Input: part model. Units: mm. Frame: model coordinates. Face numbers are marked on the shaded views. A direction names the side the tool comes from. Coordinates: 2 decimals unless noted, no trailing zeros. Order: outer loops, then holes, each group sorted by start corner. A loop starts at its lowest first (then second) coordinate and runs counter-clockwise, first axis right, second up. Notation, with made-up numbers: (-7, 33) -> (26, 33) arc R29 ccw to (26, 68) -> close; hole circle Ø7 at (14, 54.5). An arc over 180 degrees is marked (long way). Use one line per item in the form item = value. Start each with the question number.
1) Section query B-B on x = 18.5. Output: boundary loops of the cut face in (y, z).
2) Access query for the marked faces 1, 2, 3, 4 and 5. Directions: +Z, -Z, +X, -X, +Y, -Y. A direction counts if a zero-diameter tool reaches every point of the face in a straight line with its end or side. Return the directions, or none.
3) Section query D-D on y = 15.5. Output: boundary loops of the cut face in (x, z).
4) Section query C-C on y = 5. Output: boundary loops of the cut face in (x, z), then the cut area to 3 significant figures.
5) Pin query (flat end, axial travel): pin 1 (6 mm diameter, centred on x = 3.5, z = -15.5, fed in from -Y); pin 2 (3 mm diameter, centred on x = 0, y = 5, fed in from -Z); pin 3 (2 mm diameter, centred on y = 2, z = 3, fed in from +X); pin 4 (2.5 mm diameter, centred on y = 5, z = 0, fed in from +X). Return the tip coordinate at first contact, or that it passes through.
6) Ray query, line 1 along Y through (x, z) = (0, 2); line 2 along Y through (x, z) = (30.5, -28); line 3 along Z through (x, y) = (2, 5.5). Return the intervals inside material, ascending.
7) Section query A-A on z = 0. Output: boundary loops of the cut face in (x, y), then the cut area to 3 significant figures.
8) Draft query along X for the marked faces 6, 7 and 8. Return one class per face: pulls with the +X half, pulls with the -X half, needs draft (parallel to the pull), parting line crosses it, or undercut.
from build123d import *

# Parameters (mm, degrees)
SKETCH1_W           = 10
SKETCH1_H           = 10
BOSS_EXTRUDE1_DEPTH = 10
SKETCH2_R           = 1.6
CUT_EXTRUDE1_DEPTH  = 3.2
SKETCH3_R           = 1.6
CUT_EXTRUDE3_DEPTH  = 3.2
SKETCH4_R           = 1.6
CUT_EXTRUDE4_DEPTH  = 3.2
FILLET2_R           = 1
CHAMFER1_SIZE       = 6
BOSS_EXTRUDE2_DEPTH = 50
SKETCH6_R           = 1.475
CUT_EXTRUDE5_DEPTH  = 4.1
FILLET3_R           = 0.5
FILLET4_R           = 50


with BuildPart() as part:
    # Sketch1 → Boss-Extrude1 (new body)
    with BuildSketch(Plane(origin=(0, 0, 0), x_dir=(1, 0, 0), z_dir=(0, 1, 0))):
        Rectangle(SKETCH1_W, SKETCH1_H)
    extrude(amount=BOSS_EXTRUDE1_DEPTH)

    # Sketch2 → Cut-Extrude1 (cut)
    with BuildSketch(Plane.XY.offset(5)):
        with Locations((0, 5)):
            Circle(SKETCH2_R)
    extrude(amount=-CUT_EXTRUDE1_DEPTH, mode=Mode.SUBTRACT)

    # Sketch3 → Cut-Extrude3 (cut)
    with BuildSketch(Plane(origin=(0, 0, 0), x_dir=(-1, 0, 0), z_dir=(0, -1, 0))):
        with Locations(Location((0, 0, 0), (0, 0, 90))):
            Circle(SKETCH3_R)
    extrude(amount=-CUT_EXTRUDE3_DEPTH, mode=Mode.SUBTRACT)

    # Sketch4 → Cut-Extrude4 (cut)
    with BuildSketch(Plane(origin=(-5, 0, 0), x_dir=(0, 0, -1), z_dir=(1, 0, 0))):
        with Locations((0, 5)):
            Circle(SKETCH4_R)
    extrude(amount=CUT_EXTRUDE4_DEPTH, mode=Mode.SUBTRACT)

    # Fillet2
    fillet2_edges = [part.edges().sort_by_distance(p)[0] for p in [
        (0, 0, 5),
        (-5, 0, 0),
        (-5, 5, 5),
    ]]
    fillet(fillet2_edges, radius=FILLET2_R)

    # Chamfer1
    chamfer1_edges = [part.edges().sort_by_distance(p)[0] for p in [
        (5, 10, 0),
        (5, 5, -5),
        (0, 10, -5),
    ]]
    chamfer(chamfer1_edges, length=CHAMFER1_SIZE)

    # Sketch5 → Boss-Extrude2 (add)
    with BuildSketch(Plane(origin=(2.666666667, 2.666666667, -2.666666667), x_dir=(-0.4082482904638649, -0.4082482904638639, -0.8164965809277248), z_dir=(0.5773502691896257, 0.577350269189624, -0.5773502691896276))):
        Polygon((0.40824829, 4.949747468), (-2.041241452, 6.363961031), (-4.490731195, 4.949747468), (-4.490731195, 2.121320344), (-2.041241452, 0.707106781), (0.40824829, 2.121320344), align=None)
    extrude(amount=BOSS_EXTRUDE2_DEPTH)

    # Sketch13 → Loft3 section 0
    with BuildSketch(Plane(origin=(25.760677434, 25.760677434, -25.760677434), x_dir=(-0.8164965809277259, 0.4082482904638619, -0.4082482904638644), z_dir=(0.577350269189626, 0.577350269189624, -0.5773502691896274))):
        with BuildLine():
            Line((2.041241452, 6.363961031), (-0.40824829, 4.949747468))
            Line((-0.40824829, 4.949747468), (-0.40824829, 2.121320344))
            Line((-0.40824829, 2.121320344), (2.041241452, 0.707106781))
            Line((2.041241452, 0.707106781), (4.490731195, 2.121320344))
            Line((4.490731195, 2.121320344), (4.490731195, 4.949747468))
            Line((4.490731195, 4.949747468), (2.041241452, 6.363961031))
        make_face()
    # Sketch12 → Loft3 section 1
    with BuildSketch(Plane(origin=(31.534180126, 31.534180126, -31.534180126), x_dir=(-0.40824829046386485, -0.4082482904638636, -0.8164965809277249), z_dir=(0.577350269189626, 0.5773502691896241, -0.5773502691896275))):
        with BuildLine():
            Line((1.40824829, 1.543970074), (1.40824829, 5.527097737))
            Line((1.40824829, 5.527097737), (-2.041241452, 7.518661569))
            Line((-2.041241452, 7.518661569), (-5.490731195, 5.527097737))
            Line((-5.490731195, 5.527097737), (-5.490731195, 1.543970074))
            Line((-5.490731195, 1.543970074), (-2.041241452, -0.447593757))
            Line((-2.041241452, -0.447593757), (1.40824829, 1.543970074))
        make_face()
    loft()

    # Sketch6 → Cut-Extrude5 (cut)
    with BuildSketch(Plane(origin=(31.534180126, 31.534180126, -31.534180126), x_dir=(-0.40824829046386507, -0.4082482904638639, -0.8164965809277246), z_dir=(0.5773502691896257, 0.5773502691896238, -0.5773502691896278))):
        with Locations(Location((-2.041241452, 3.535533906, 0), (0, 0, 30))):
            Circle(SKETCH6_R)
    extrude(amount=-CUT_EXTRUDE5_DEPTH, mode=Mode.SUBTRACT)

    # Fillet3
    fillet3_edges = [part.edges().sort_by_distance(p)[0] for p in [
        (28.459265169, 37.68401004, -28.459265169),
        (31.27576175, 36.27576175, -27.051016879),
        (32.68401004, 33.459265169, -28.459265169),
        (31.27576175, 32.051016879, -31.27576175),
        (28.459265169, 33.459265169, -32.68401004),
        (27.051016879, 36.27576175, -31.27576175),
    ]]
    fillet(fillet3_edges, radius=FILLET3_R)

    # Fillet4
    # the kernel refuses this fillet: 50 mm, written as the material it adds along each edge
    with BuildSketch(Plane(origin=(30.502434506, 27.094010768, -19.685587029), x_dir=(0.6151072128065446, 0.49324054325118827, -0.6151072128065457), z_dir=(-0.7071067811865475, -1.8318679906315083e-15, -0.7071067811865477))) as fillet4_piece_1_section:
        with BuildLine():
            CenterArc((FILLET4_R * 0.0498756211209, FILLET4_R), FILLET4_R, 264.289406863, 5.710593137)
            Line((-FILLET4_R * 0.0496280979001, FILLET4_R * 0.00496280979001), (0, 0))
            Line((0, 0), (FILLET4_R * 0.0498756211209, 0))
        make_face()
    fillet4_piece_1 = extrude(amount=15.297332405, mode=Mode.PRIVATE)
    fillet4_piece_1 = fillet4_piece_1 - Plane(origin=(5.44602295, 2.037599211, -65.47905465), x_dir=(0.4636707308133369, 0.463670730813339, 0.7549959647402431), z_dir=(0.7071067811865475, -0.7071067811865478, 2.220446049250313e-15)) * Cylinder(50, 41, mode=Mode.PRIVATE)
    fillet4_piece_1 = fillet4_piece_1 - Plane(origin=(65.47905465, 7.44602295, -0.037599211), x_dir=(-0.7549959647402456, 0.4636707308133344, -0.46367073081333715), z_dir=(0, 0.7071067811865497, 0.7071067811865455)) * Cylinder(50, 41, mode=Mode.PRIVATE)
    add(fillet4_piece_1)
    with BuildSketch(Plane(origin=(26.094010768, 33.502434506, -17.685587029), x_dir=(0.6557294359916664, 0.5338627664363041, -0.5338627664363074), z_dir=(0, -0.7071067811865497, -0.7071067811865455))) as fillet4_piece_2_section:
        with BuildLine():
            CenterArc((FILLET4_R * 0.0498756211209, FILLET4_R), FILLET4_R, 264.289406863, 5.710593137)
            Line((-FILLET4_R * 0.0496280979001, FILLET4_R * 0.00496280979001), (0, 0))
            Line((0, 0), (FILLET4_R * 0.0498756211209, 0))
        make_face()
    fillet4_piece_2 = extrude(amount=15.297332405, mode=Mode.PRIVATE)
    fillet4_piece_2 = fillet4_piece_2 - Plane(origin=(42.862428257, 50.270851996, 20.170603443), x_dir=(-0.3487737328890522, -0.34877373288905417, -0.8698929626645284), z_dir=(-0.7071067811865471, 0.7071067811865479, -1.8596235662471372e-15)) * Cylinder(50, 41, mode=Mode.PRIVATE)
    fillet4_piece_2 = fillet4_piece_2 - Plane(origin=(48.270851996, -15.170603443, -39.862428257), x_dir=(-0.34877373288905117, 0.8698929626645311, 0.3487737328890489), z_dir=(0.7071067811865476, 1.831867990631508e-15, 0.7071067811865476)) * Cylinder(50, 41, mode=Mode.PRIVATE)
    add(fillet4_piece_2)
    with BuildSketch(Plane(origin=(19.685587029, 35.502434506, -22.094010768), x_dir=(0.6151072128065466, 0.6151072128065448, -0.49324054325118677), z_dir=(0.7071067811865472, -0.7071067811865479, 1.7763568394002505e-15))) as fillet4_piece_3_section:
        with BuildLine():
            CenterArc((FILLET4_R * 0.0498756211209, FILLET4_R), FILLET4_R, 264.289406863, 5.710593137)
            Line((-FILLET4_R * 0.0496280979001, FILLET4_R * 0.00496280979001), (0, 0))
            Line((0, 0), (FILLET4_R * 0.0498756211209, 0))
        make_face()
    fillet4_piece_3 = extrude(amount=15.297332405, mode=Mode.PRIVATE)
    fillet4_piece_3 = fillet4_piece_3 - Plane(origin=(0.037599211, 70.47905465, -2.44602295), x_dir=(0.46367073081333604, -0.7549959647402467, -0.4636707308133341), z_dir=(-0.7071067811865476, -1.6930901125533633e-15, -0.7071067811865477)) * Cylinder(50, 41, mode=Mode.PRIVATE)
    fillet4_piece_3 = fillet4_piece_3 - Plane(origin=(65.47905465, 10.44602295, 2.962400789), x_dir=(-0.7549959647402456, 0.4636707308133344, -0.46367073081333715), z_dir=(0, 0.7071067811865497, 0.7071067811865455)) * Cylinder(50, 41, mode=Mode.PRIVATE)
    add(fillet4_piece_3)
    with BuildSketch(Plane(origin=(17.685587029, 31.094010768, -28.502434506), x_dir=(0.533862766436308, 0.6557294359916612, -0.5338627664363096), z_dir=(0.7071067811865475, 1.7763568394002505e-15, 0.7071067811865476))) as fillet4_piece_4_section:
        with BuildLine():
            CenterArc((FILLET4_R * 0.0498756211209, FILLET4_R), FILLET4_R, 264.289406863, 5.710593137)
            Line((-FILLET4_R * 0.0496280979001, FILLET4_R * 0.00496280979001), (0, 0))
            Line((0, 0), (FILLET4_R * 0.0498756211209, 0))
        make_face()
    fillet4_piece_4 = extrude(amount=15.297332405, mode=Mode.PRIVATE)
    fillet4_piece_4 = fillet4_piece_4 - Plane(origin=(39.862428257, 53.270851996, 20.170603443), x_dir=(-0.3487737328890522, -0.34877373288905417, -0.8698929626645284), z_dir=(-0.7071067811865471, 0.7071067811865479, -1.8596235662471372e-15)) * Cylinder(50, 41, mode=Mode.PRIVATE)
    fillet4_piece_4 = fillet4_piece_4 - Plane(origin=(-20.170603443, 47.862428257, -45.270851996), x_dir=(0.8698929626645304, -0.34877373288904956, 0.3487737328890521), z_dir=(0, -0.7071067811865497, -0.7071067811865454)) * Cylinder(50, 41, mode=Mode.PRIVATE)
    add(fillet4_piece_4)
    with BuildSketch(Plane(origin=(28.502434506, 22.685587029, -26.094010768), x_dir=(0.5338627664363049, 0.5338627664363026, -0.6557294359916698), z_dir=(-0.7071067811865474, 0.7071067811865477, -2.220446049250313e-15))) as fillet4_piece_5_section:
        with BuildLine():
            CenterArc((FILLET4_R * 0.0498756211209, FILLET4_R), FILLET4_R, 264.289406863, 5.710593137)
            Line((-FILLET4_R * 0.0496280979001, FILLET4_R * 0.00496280979001), (0, 0))
            Line((0, 0), (FILLET4_R * 0.0498756211209, 0))
        make_face()
    fillet4_piece_5 = extrude(amount=15.297332405, mode=Mode.PRIVATE)
    fillet4_piece_5 = fillet4_piece_5 - Plane(origin=(45.270851996, -15.170603443, -42.862428257), x_dir=(-0.34877373288905117, 0.8698929626645311, 0.3487737328890489), z_dir=(0.7071067811865476, 1.831867990631508e-15, 0.7071067811865476)) * Cylinder(50, 41, mode=Mode.PRIVATE)
    fillet4_piece_5 = fillet4_piece_5 - Plane(origin=(-20.170603443, 44.862428257, -48.270851996), x_dir=(0.8698929626645304, -0.34877373288904956, 0.3487737328890521), z_dir=(0, -0.7071067811865497, -0.7071067811865454)) * Cylinder(50, 41, mode=Mode.PRIVATE)
    add(fillet4_piece_5)
    with BuildSketch(Plane(origin=(22.094010768, 24.685587029, -30.502434506), x_dir=(0.49324054325118744, 0.6151072128065436, -0.6151072128065473), z_dir=(0, 0.7071067811865498, 0.7071067811865454))) as fillet4_piece_6_section:
        with BuildLine():
            CenterArc((FILLET4_R * 0.0498756211209, FILLET4_R), FILLET4_R, 264.289406863, 5.710593137)
            Line((-FILLET4_R * 0.0496280979001, FILLET4_R * 0.00496280979001), (0, 0))
            Line((0, 0), (FILLET4_R * 0.0498756211209, 0))
        make_face()
    fillet4_piece_6 = extrude(amount=15.297332405, mode=Mode.PRIVATE)
    fillet4_piece_6 = fillet4_piece_6 - Plane(origin=(2.44602295, 5.037599211, -65.47905465), x_dir=(0.4636707308133369, 0.463670730813339, 0.7549959647402431), z_dir=(0.7071067811865475, -0.7071067811865478, 2.220446049250313e-15)) * Cylinder(50, 41, mode=Mode.PRIVATE)
    fillet4_piece_6 = fillet4_piece_6 - Plane(origin=(-2.962400789, 70.47905465, -5.44602295), x_dir=(0.46367073081333604, -0.7549959647402467, -0.4636707308133341), z_dir=(-0.7071067811865476, -1.6930901125533633e-15, -0.7071067811865477)) * Cylinder(50, 41, mode=Mode.PRIVATE)
    add(fillet4_piece_6)


solid = part.part
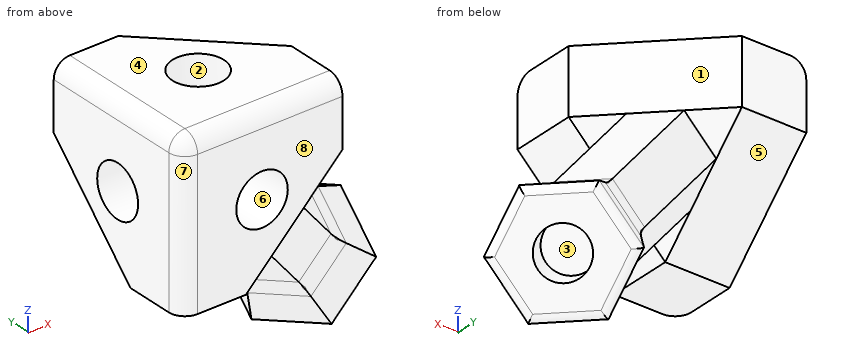
Answers below:
q1.outline = (19.5, -16.5) -> (21.5, -20.5) -> (25.5, -22.5) -> (27.5, -20.5) -> (25.5, -16.5) -> (21.5, -14.5) -> close
q2.face_1 = +Z, +X, +Y
q2.face_2 = +Z
q2.face_3 = none
q2.face_4 = +Z, +X, -X, +Y, -Y
q2.face_5 = -Z, -X, +Y
q3.outline = (6.5, -8.5) -> (8.5, -12.5) -> (12.5, -14.5) -> (14.5, -12.5) -> (12.5, -8.5) -> (8.5, -6.5) -> close
q4.outline = (-5, -4) -> (-1, -4) -> (0, -3) -> (2, -4) -> (4, -2) -> (3, 0) -> (4, 1) -> (4, 5) -> (1.6, 5) -> (1.6, 1.8) -> (-1.6, 1.8) -> (-1.6, 5) -> (-4, 5) arc R1 ccw to (-5, 4) -> (-5, 1.6) -> (-1.8, 1.6) -> (-1.8, -1.6) -> (-5, -1.6) -> close
q4.area = 55.3 mm^2
q5.pin_1 = through
q5.pin_2 = -5
q5.pin_3 = 5
q5.pin_4 = 4.77
q6.line_1 = 0 to 3.4, 6.6 to 9
q6.line_2 = 30.43 to 36.1
q6.line_3 = -4.25 to 5
q7.outline = (-5, 1) arc R1 ccw to (-4, 0) -> (-1.6, 0) -> (-1.6, 3.2) -> (1.6, 3.2) -> (1.6, 0) -> (4, 0) -> (4, 4) -> (3, 5) -> (4, 7) -> (2, 9) -> (0, 8) -> (-1, 9) -> (-5, 9) -> (-5, 6.6) -> (-1.8, 6.6) -> (-1.8, 3.4) -> (-5, 3.4) -> close
q7.area = 55.3 mm^2
q8.face_6 = undercut
q8.face_7 = pulls with the -X half
q8.face_8 = needs draft
